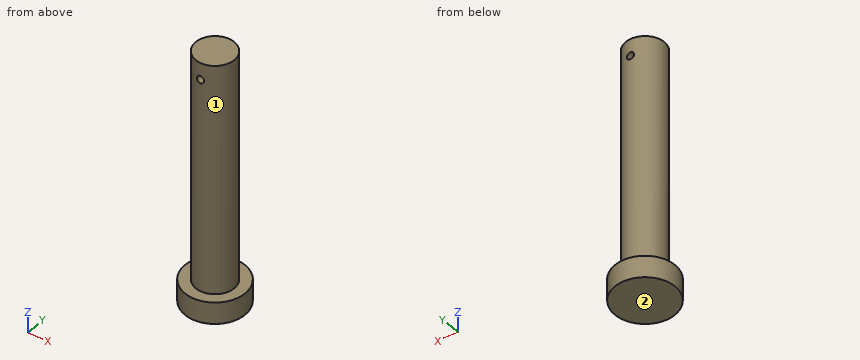
Solid Edge part; units mm, degrees
sketch "Sketch1" plane through (0, 0, 0) normal (0, 0, 1) x (1, 0, 0)
  circle A0 centre (0, 0) radius 12.5
extrude "Protrusion1" add sketch "Sketch1" along normal blind 9
sketch "Sketch2" plane through (0, 0, 9) normal (0, 0, 1) x (1, 0, 0)
  circle A0 centre (0, 0) radius 8
extrude "ExtrudedProtrusion_2" add sketch "Sketch2" along normal blind 96
sketch "Sketch3" plane through (0, 0, 0) normal (0, -1, 0) x (1, 0, 0)
  circle A0 centre (0, 98) radius 1.5
extrude "ExtrudedCutout_1" cut sketch "Sketch3" along normal mid plane 130.3633
properties part number "5" material "Fe - 410 W"
Build history of the part. All positions in model axes, mm. Face numbers are marked on the shaded views. A direction names the side the tool comes from. Coordinates: 2 decimals unless noted, no trailing zeros. Write each loop counter-clockwise with the first axis right and the second up, starting at its lowest first coordinate (ties: lowest second). Pieces come first, ordered by that corner, then holes.
1. Drill centre lines: probe 1 along Z at (x, y) = (0, 0.75); probe 2 along X at (y, z) = (-0.25, 98); probe 3 along Z at (x, y) = (-2, 9). Where is each one in solid material? Low to high.
Answer block:
probe 1: z = 0 to 96.5, 99.5 to 105
probe 2: x = -8 to -1.5, 1.5 to 8
probe 3: z = 0 to 9
2. 3-axis set-ups, long thin cutter, end or side, ignore diameter. For the marked faces 1 and 2: which of +Z, -Z, +X, -X, +Y, -Y reach the whole face in a straight line?
Answer block:
face 1: +Z
face 2: -Z, +X, -X, +Y, -Y
3. Drop flat-ended pins along their axis: pin 1 (2 mm diameter, centred on y = -6, z = 66, fed in from +X) (3 decimals); pin 2 (10 mm diameter, centred on x = 0, z = 42, fed in from -Y); pin 3 (4 mm diameter, centred on x = 0, z = 98, fed in from +Y). Give the stop position or say it passes through.
Answer block:
pin 1: stops at x = 6.245
pin 2: stops at y = -8
pin 3: stops at y = 8
4. Band-saw the part on C-C, the plane z = 98. Give the cut face in (x, y), and give its area (3 significant figures).
Answer block:
outline: (-1.5, -7.86) - (-1.5, 7.86) arc R8 ccw to start; (1.5, -7.86) arc R8 ccw to (1.5, 7.86) - close
area: 153 mm2
5. Band-saw the part on D-D, the plane x = -6.75. Give the cut face in (y, z), and give its area (3 significant figures).
Answer block:
outline: (-10.52, 0) - (10.52, 0) - (10.52, 9) - (4.29, 9) - (4.29, 105) - (-4.29, 105) - (-4.29, 9) - (-10.52, 9) - close
area: 1,010 mm2
6. Band-saw the part on A-A, the plane x = 0. Give the cut face in (y, z).
Answer block:
outline: (-12.5, 0) - (12.5, 0) - (12.5, 9) - (8, 9) - (8, 96.5) - (-8, 96.5) - (-8, 9) - (-12.5, 9) - close; (-8, 99.5) - (8, 99.5) - (8, 105) - (-8, 105) - close
7. Band-saw the part on B-B, the plane y = 0. Give the cut face in (x, z).
Answer block:
outline: (-12.5, 0) - (12.5, 0) - (12.5, 9) - (8, 9) - (8, 105) - (-8, 105) - (-8, 9) - (-12.5, 9) - close; hole circle Ø3 at (0, 98)
